```python
from build123d import *

# Parameters (mm, degrees)
SKETCH_1_W          = 91
SKETCH_1_H          = 45
EXTRUDE_1_DEPTH     = 1.6
SKETCH_2_R          = 1.3
CUT_EXTRUDE_1_DEPTH = 1.6
SKETCH_5_W          = 10
SKETCH_5_H          = 6.5
CUT_EXTRUDE_2_DEPTH = 1.6


with BuildPart() as part:
    # Эскиз1 → Бобышка-Вытянуть1 (new body)
    with BuildSketch(Plane.XY):
        Rectangle(SKETCH_1_W, SKETCH_1_H)
    extrude(amount=EXTRUDE_1_DEPTH)

    # Эскиз2 → Вырез-Вытянуть1 (cut)
    with BuildSketch(Plane(origin=(0, 0, 0), x_dir=(-1, 0, 0), z_dir=(0, 0, -1))):
        with Locations((22, 20)):
            Circle(SKETCH_2_R)
        with Locations((-22, 20)):
            Circle(SKETCH_2_R)
        with Locations((42, 20)):
            Circle(SKETCH_2_R)
        with Locations((42, -20)):
            Circle(SKETCH_2_R)
        with Locations((22, -20)):
            Circle(SKETCH_2_R)
        with Locations((-22, -20)):
            Circle(SKETCH_2_R)
    extrude(amount=-CUT_EXTRUDE_1_DEPTH, mode=Mode.SUBTRACT)

    # Эскиз5 → Вырез-Вытянуть2 (cut)
    with BuildSketch(Plane(origin=(0, 0, 0), x_dir=(-1, 0, 0), z_dir=(0, 0, -1))):
        with Locations((-32, 19.25)):
            Rectangle(SKETCH_5_W, SKETCH_5_H)
        with Locations((32, 19.25)):
            Rectangle(SKETCH_5_W, SKETCH_5_H)
        with Locations((32, -19.25)):
            Rectangle(SKETCH_5_W, SKETCH_5_H)
        with Locations((-32, -19.25)):
            Rectangle(SKETCH_5_W, SKETCH_5_H)
    extrude(amount=-CUT_EXTRUDE_2_DEPTH, mode=Mode.SUBTRACT)


solid = part.part
```
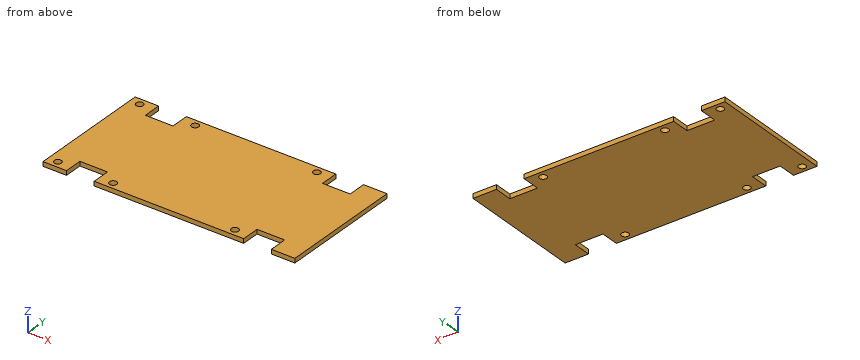
Can you work these out from the model? Positions are in its coordinate system, mm. Coordinates: 2 decimals unless noted, no trailing zeros. Loops run counter-clockwise (first coordinate to the right, second up) from the corner with the lowest first, then second, coordinate; pieces in that order, holes last. Notation, with made-up numbers: (-2.75, -12.5) -> (48.25, -12.5) arc R23 cw to (48.25, 12.5) -> close; hole circle Ø6 at (70, 34.25). An arc over 180 degrees is marked (long way). Answer as a JSON object with one key per item and string values.
1) If I drill on line 1 (Y direction, x = -22, z = 1); line 2 (X direction, y = -18, z = 1.35); line 3 (X direction, y = 19.5, z = 0.35), over which ranges is the centre line in solid material (lowest first)?
Results:
{"line 1": "y = -22.5 to -21.3, -18.7 to 18.7, 21.3 to 22.5", "line 2": "x = -45.5 to -37, -27 to 27, 37 to 45.5", "line 3": "x = -45.5 to -43.2, -40.8 to -37, -27 to -23.2, -20.8 to 20.8, 23.2 to 27, 37 to 45.5"}
2) For P1, Ø1.6, axis at x = -22, y = -20, coming from the +Z side, with a flat end and sliding along its axis, tell me the tip position at first contact or that it passes through.
Results:
{"P1": "passes through"}
3) Imagine slicing it at B-B (y = 20). Please give me the cut outline in (x, z), then the cut area to 3 significant figures.
Results:
{"outline": "(-45.5, 0) -> (-43.3, 0) -> (-43.3, 1.6) -> (-45.5, 1.6) -> close; (-40.7, 0) -> (-37, 0) -> (-37, 1.6) -> (-40.7, 1.6) -> close; (-27, 0) -> (-23.3, 0) -> (-23.3, 1.6) -> (-27, 1.6) -> close; (-20.7, 0) -> (20.7, 0) -> (20.7, 1.6) -> (-20.7, 1.6) -> close; (23.3, 0) -> (27, 0) -> (27, 1.6) -> (23.3, 1.6) -> close; (37, 0) -> (45.5, 0) -> (45.5, 1.6) -> (37, 1.6) -> close", "area": "101 mm^2"}
4) Imagine slicing it at C-C (z = 0.8). Please give me the cut outline in (x, y), then the cut area to 3 significant figures.
Results:
{"outline": "(-45.5, -22.5) -> (-37, -22.5) -> (-37, -16) -> (-27, -16) -> (-27, -22.5) -> (27, -22.5) -> (27, -16) -> (37, -16) -> (37, -22.5) -> (45.5, -22.5) -> (45.5, 22.5) -> (37, 22.5) -> (37, 16) -> (27, 16) -> (27, 22.5) -> (-27, 22.5) -> (-27, 16) -> (-37, 16) -> (-37, 22.5) -> (-45.5, 22.5) -> close; hole circle Ø2.6 at (-42, -20); hole circle Ø2.6 at (-42, 20); hole circle Ø2.6 at (-22, -20); hole circle Ø2.6 at (-22, 20); hole circle Ø2.6 at (22, -20); hole circle Ø2.6 at (22, 20)", "area": "3,800 mm^2"}
5) Imagine slicing it at A-A (x = -22). Please give me the cut outline in (y, z), then the cut area to 3 significant figures.
Results:
{"outline": "(-22.5, 0) -> (-21.3, 0) -> (-21.3, 1.6) -> (-22.5, 1.6) -> close; (-18.7, 0) -> (18.7, 0) -> (18.7, 1.6) -> (-18.7, 1.6) -> close; (21.3, 0) -> (22.5, 0) -> (22.5, 1.6) -> (21.3, 1.6) -> close", "area": "63.7 mm^2"}
